from build123d import *

# Parameters (mm, degrees)
BOSS_EXTRUDE1_DEPTH     = 1190
CUT_EXTRUDE1_DEPTH      = 1191.176063656
CUT_EXTRUDE1_DEPTH_BACK = 1191.176063656


with BuildPart() as part:
    # Sketch1 → Boss-Extrude1 (new body)
    with BuildSketch(Plane.XY):
        Polygon((-9.75, -9.75), (9.75, -9.75), (9.75, -8.25), (0.75, -8.25), (0.75, 9.75), (-0.75, 9.75), (-0.75, -8.25), (-9.75, -8.25), align=None)
    extrude(amount=BOSS_EXTRUDE1_DEPTH)

    # Sketch2 → Cut-Extrude1 (cut, two sides: drawn at the far end of the back side and taken through both)
    with BuildSketch(Plane(origin=(0, -8.25, 0), x_dir=(1, 0, 0), z_dir=(0, 1, 0)).offset(-CUT_EXTRUDE1_DEPTH_BACK)):
        Polygon((9.75, 0), (-9.75, -19.5), (-15.874453794, -19.5), (-15.874453794, 8.440692937), (9.75, 8.440692937), align=None)
        Polygon((9.75, -1190), (-9.75, -1170.5), (-13.500903001, -1170.5), (-13.500903001, -1195.414043503), (9.75, -1195.414043503), align=None)
    extrude(amount=CUT_EXTRUDE1_DEPTH + CUT_EXTRUDE1_DEPTH_BACK, mode=Mode.SUBTRACT)


solid = part.part
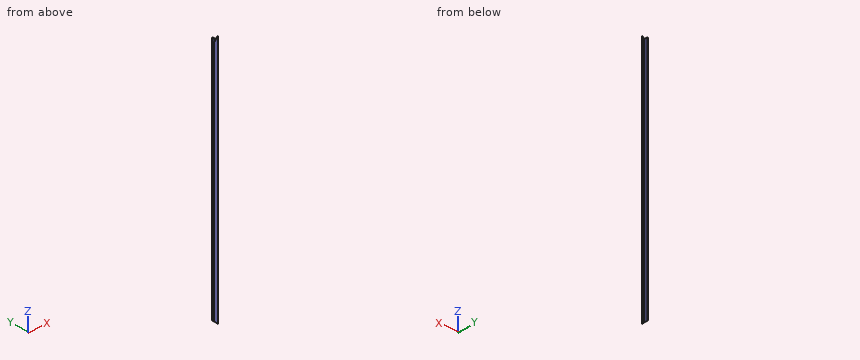
Can you work these out from the model? Positions are in its coordinate system, mm. Coordinates: 2 decimals unless noted, no trailing zeros. Loops run counter-clockwise (first coordinate to the right, second up) from the corner with the lowest first, then second, coordinate; pieces in that order, holes last. Notation, with made-up numbers: (59, 21) - (118, 21) arc R22 cw to (118, 34) - close; hole circle Ø9 at (65, 35.5). An arc over 180 degrees is marked (long way). Answer as a JSON object with one key per item and string values. Group by question number.
Item 1: If we section it at A-A (z = 195): List the corners of the cut face in (x, y) for me.
Item 2: For pin 1 (1.5 mm diameter, centred on y = -5.5, z = 607, fed in from -X); pin 2 (2.5 mm diameter, centred on x = 7, z = 353, fed in from +Y), each with a flat end and sliding along its axis, tell me the tip position at first contact or that it passes through.
Item 3: If I drill on L1, parallel to Y at x = -2, z = 904; L2, parallel to X at y = 0.5, z = 630.5, over which ranges is the centre line in solid material (lowest first)? Write a range as from..to.
Item 4: If we section it at B-B (x = -4.5): List the corners of the cut face in (y, z) for me, plus the area to 3 significant figures.
Item 5: If we section it at C-C (y = 5.5): List the corners of the cut face in (x, z) for me, plus the area to 3 significant figures.
Returned:
{
 "1": {"outline": "(-9.75, -9.75) - (9.75, -9.75) - (9.75, -8.25) - (0.75, -8.25) - (0.75, 9.75) - (-0.75, 9.75) - (-0.75, -8.25) - (-9.75, -8.25) - close"},
 "2": {"pin 1": "stops at x = -0.75", "pin 2": "stops at y = -8.25"},
 "3": {"L1": "y = -9.75..-8.25", "L2": "x = -0.75..0.75"},
 "4": {"outline": "(-9.75, 14.25) - (-8.25, 14.25) - (-8.25, 1175.75) - (-9.75, 1175.75) - close", "area": "1,740 mm²"},
 "5": {"outline": "(-0.75, 10.5) - (0.75, 9) - (0.75, 1181) - (-0.75, 1179.5) - close", "area": "1,760 mm²"}
}
